Can you work these out from the model? Positions are in its coordinate system, mm. A direction names the side the tool comes from. Coordinates: 2 decimals unless noted, no trailing zeros. Order: outer loops, then holes, each group sorted by start corner. A loop starts at its lowest first (then second) coordinate and runs counter-clockwise, first axis right, second up. Notation, with made-up numbers: (-35, 89.25) -> (-16, 89.25) arc R8 cw to (-16, 101.25) -> close; hole circle Ø5 at (78, 42). An arc over 180 degrees is marked (long way). Answer as CSV lines item,"result".
from build123d import *

# Parameters (mm, degrees)
SALIENTE_EXTRUIR1_DEPTH = 4
SALIENTE_EXTRUIR2_DEPTH = 35


with BuildPart() as part:
    # Croquis1 → Saliente-Extruir1 (new body)
    with BuildSketch(Plane(origin=(0, 0, 0), x_dir=(1, 0, 0), z_dir=(0, 1, 0))):
        Polygon((8.284271247, 28.284271247), (36.568542495, 0), (8.284271247, -28.284271247), (-20, 0), align=None)
    extrude(amount=SALIENTE_EXTRUIR1_DEPTH)

    # Croquis2 → Saliente-Extruir2 (add)
    with BuildSketch(Plane(origin=(0, 4, 0), x_dir=(1, 0, 0), z_dir=(0, 1, 0))):
        Polygon((-20, 0), (-16.464466094, 3.535533906), (8.284271247, -21.213203436), (33.033008589, 3.535533906), (36.568542495, 0), (8.284271247, -28.284271247), align=None)
    extrude(amount=SALIENTE_EXTRUIR2_DEPTH)


solid = part.part
Q1. Which directions (+Z, -Z, +X, -X, +Y, -Y) give clear straight access to the entire face, cutting with the end or side of a thin tool? Please do faces 4 (the flat face through (13, 39, 17)), 5 (the flat face through (-4.26, 21.26, 8.67)).
Solution:
face 4,"+Z, -Z, +X, -X, +Y"
face 5,"-Z, +Y"
Q2. Imagine slicing it at D-D (z = -19). List the corners of the cut face in (x, y) for me.
Solution:
outline,"(-1, 0) -> (17.57, 0) -> (17.57, 4) -> (-1, 4) -> close"
Q3. If I drill on line 1 (Y direction, x = 12, z = 6); line 2 (X direction, y = 34, z = 7.5); line 3 (X direction, y = 6, z = -0.5), over which ranges is the centre line in solid material (lowest first)?
Solution:
line 1,"0 to 4"
line 2,"-12.5 to -5.43, 22 to 29.07"
line 3,"-19.5 to -13.43, 30 to 36.07"
Q4. Imagine slicing it at C-C (x = 31.5). List the corners of the cut face in (y, z) for me.
Solution:
outline,"(0, -5.07) -> (4, -5.07) -> (4, -2) -> (39, -2) -> (39, 5.07) -> (0, 5.07) -> close"
Q5. Imagine slicing it at B-B (z = 8). List the corners of the cut face in (x, y) for me.
Solution:
outline,"(-12, 0) -> (28.57, 0) -> (28.57, 39) -> (21.5, 39) -> (21.5, 4) -> (-4.93, 4) -> (-4.93, 39) -> (-12, 39) -> close"
Q6. We'd pull the mould along X, two halves only. Please class faces 1 (the flat face through (9, 4, -4)), 2 (the flat face through (9, 0, 0)), 3 (the flat face through (-6, 19, 14)): pulls with the +X half, pulls with the -X half, needs draft (parallel to the pull), parting line crosses it, or undercut.
Solution:
face 1,"undercut"
face 2,"needs draft"
face 3,"pulls with the -X half"
Q7. Imagine slicing it at A-A (y = 24). List the corners of the cut face in (x, z) for me, and give its area (3 significant figures).
Solution:
outline,"(-20, 0) -> (-16.46, -3.54) -> (8.28, 21.21) -> (33.03, -3.54) -> (36.57, 0) -> (8.28, 28.28) -> close"
area,"375 mm2"
Q8. For P1, Ø6, axis at x = 25.5, z = -13, coming from the +Y side; P2, Ø1, axis at x = 12.5, y = 16, coming from the +Z side; P3, Ø10, axis at y = 26, z = 6, coming from the +X side, each with a flat end and sliding along its axis, tell me the tip position at first contact or that it passes through.
Solution:
P1,"y = 4"
P2,"z = 24.57"
P3,"x = 35.57"
